```python
from build123d import *

# Parameters (mm, degrees)
SKETCH1_W           = 406.4
SKETCH1_H           = 50.8
BOSS_EXTRUDE1_DEPTH = 6.35
CUT_EXTRUDE1_DEPTH  = 6.35
FILLET1_R           = 6.35
SKETCH3_R           = 3.175
CUT_EXTRUDE2_DEPTH  = 6.35
FILLET3_R           = 3.175


with BuildPart() as part:
    # Sketch1 → Boss-Extrude1 (new body)
    with BuildSketch(Plane.XY):
        Rectangle(SKETCH1_W, SKETCH1_H)
    extrude(amount=BOSS_EXTRUDE1_DEPTH)

    # Sketch2 → Cut-Extrude1 (cut)
    with BuildSketch(Plane.XY.offset(6.35)):
        with BuildLine():
            Line((-88.9, -15.875), (88.9, -15.875))
            ThreePointArc((88.9, -15.875), (93.390128061, -14.015128061), (95.25, -9.525))
            Line((95.25, -9.525), (95.25, 9.525))
            ThreePointArc((95.25, 9.525), (93.390128061, 14.015128061), (88.9, 15.875))
            Line((88.9, 15.875), (-88.9, 15.875))
            ThreePointArc((-88.9, 15.875), (-93.390128061, 14.015128061), (-95.25, 9.525))
            Line((-95.25, 9.525), (-95.25, -9.525))
            ThreePointArc((-95.25, -9.525), (-93.390128061, -14.015128061), (-88.9, -15.875))
        make_face()
    extrude(amount=-CUT_EXTRUDE1_DEPTH, mode=Mode.SUBTRACT)

    # Fillet1
    fillet1_edges = [part.edges().sort_by_distance(p)[0] for p in [
        (203.2, -25.4, 3.175),
        (-203.2, -25.4, 3.175),
        (-203.2, 25.4, 3.175),
        (203.2, 25.4, 3.175),
    ]]
    fillet(fillet1_edges, radius=FILLET1_R)

    # Sketch3 → Cut-Extrude2 (cut)
    with BuildSketch(Plane.XY.offset(6.35)):
        with Locations((-190.5, 12.7)):
            Circle(SKETCH3_R)
        with Locations((-190.5, -12.7)):
            Circle(SKETCH3_R)
        with Locations(Location((190.5, -12.7, 0), (0, 0, 180))):
            Circle(SKETCH3_R)
        with Locations(Location((190.5, 12.7, 0), (0, 0, 180))):
            Circle(SKETCH3_R)
    extrude(amount=-CUT_EXTRUDE2_DEPTH, mode=Mode.SUBTRACT)

    # Fillet3
    fillet3_edges = [part.edges().sort_by_distance(p)[0] for p in [
        (-93.390128061, -14.015128061, 0),
        (-95.25, 0, 0),
        (-93.390128061, 14.015128061, 0),
        (0, 15.875, 0),
        (93.390128061, 14.015128061, 0),
        (95.25, 0, 0),
        (93.390128061, -14.015128061, 0),
        (-93.390128061, -14.015128061, 6.35),
        (-95.25, 0, 6.35),
        (-93.390128061, 14.015128061, 6.35),
        (0, 15.875, 6.35),
        (93.390128061, 14.015128061, 6.35),
        (95.25, 0, 6.35),
        (93.390128061, -14.015128061, 6.35),
        (0, -15.875, 0),
        (0, -15.875, 6.35),
    ]]
    fillet(fillet3_edges, radius=FILLET3_R - 0.0001)  # a hair under: the kernel refuses the full size


solid = part.part
```
Input: part model. Units: mm. Frame: model coordinates. Round coordinates to 2 decimals unless told otherwise and drop trailing zeros. Loops run counter-clockwise (first coordinate to the right, second up) from the corner with the lowest first, then second, coordinate; pieces in that order, holes last.
1) Section query B-B on z = 5. Return the cut outline in (x, y) (3 decimals), plus the area to 3 significant figures.
Ans:
outline: (-203.2, -19.05) arc R6.35 ccw to (-196.85, -25.4) - (196.85, -25.4) arc R6.35 ccw to (203.2, -19.05) - (203.2, 19.05) arc R6.35 ccw to (196.85, 25.4) - (-196.85, 25.4) arc R6.35 ccw to (-203.2, 19.05) - close; hole circle Ø6.35 at (-190.5, -12.7); hole circle Ø6.35 at (-190.5, 12.7); hole (-95.827, -9.525) arc R6.927 ccw to (-88.9, -16.452) - (88.9, -16.452) arc R6.927 ccw to (95.827, -9.525) - (95.827, 9.525) arc R6.927 ccw to (88.9, 16.452) - (-88.9, 16.452) arc R6.927 ccw to (-95.827, 9.525) - close; hole circle Ø6.35 at (190.5, -12.7); hole circle Ø6.35 at (190.5, 12.7)
area: 14,200 mm2
2) Material intervals for line 1 (Y direction, x = -190.5, z = 3.75) (3 decimals); line 2 (Y direction, x = 19, z = 3.5); line 3 (X direction, y = -13, z = 4.75), sorted ascending.
Ans:
line 1: y = -25.4 to -15.875, -9.525 to 9.525, 15.875 to 25.4
line 2: y = -25.4 to -15.89, 15.89 to 25.4
line 3: x = -203.2 to -193.66, -187.34 to -94.71, 94.71 to 187.34, 193.66 to 203.2
3) Pull-direction query (Y, two-part tool) for faces 1 (the cylindrical face through (201.29, -23.59, 3.22)), 2 (the cylindrical face through (-193.67, -12.56, 3.22)), 3 (the cylindrical face through (201.29, 23.59, 3.22)); classes: released by +Y, released by -Y, zero draft, split by the parting line, or undercut.
Ans:
face 1: released by -Y
face 2: undercut
face 3: released by +Y
